For this review, use the dimensioned drawing (mm, ordinates from the lowest corner) and the shaded views. Round coordinates to 2 decimals unless told otherwise and drop trailing zeros. Order: outer loops, then holes, each group sorted by start corner. A loop starts at its lowest first (then second) coordinate and runs counter-clockwise, first axis right, second up. Notation, with made-up numbers: (-5, -36) - (14, -36) arc R21 ccw to (14, -24) - close; hole circle Ø1 at (46, 28.25). An arc over 180 degrees is marked (long way). Write item = value, one per line.
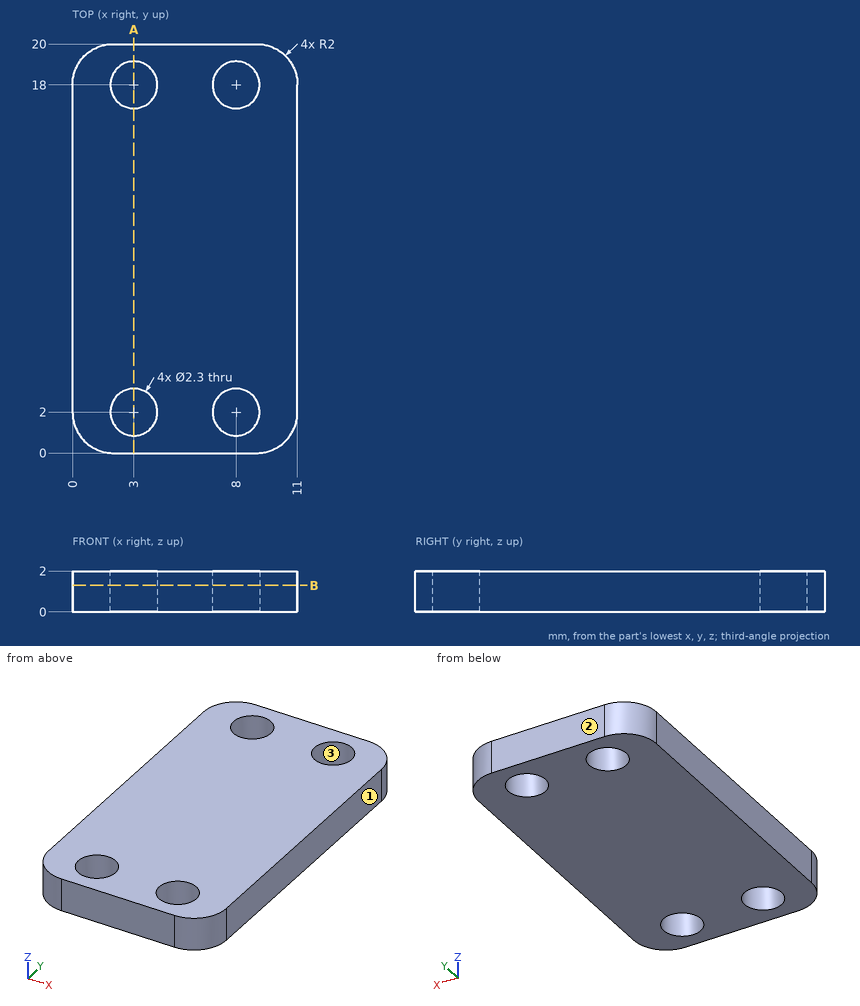
1) Clearance check with a flat-ended pin moving along its axis: pin 1 Ø1.8 at (x, y) = (8, 2) entering from +Z. State where the tip first meets the part, or that it passes through.
Findings:
pin_1 = through
2) To check wall thickness, follow L1, parallel to Y at x = 8, z = 0.8; L2, parallel to Y at x = 2.25, z = 0.1; L3, parallel to X at y = 1.5, z = 0.75. State the ranges of each line that lie inside material, in increasing order. Write a range as from..to.
Findings:
L1 = 0..0.85, 3.15..16.85, 19.15..20
L2 = 0..1.13, 2.87..17.13, 18.87..20
L3 = 0.06..1.96, 4.04..6.96, 9.04..10.94
3) The part is to be moulded in two halves that separate along Y. For the marked faces 1, 2 and 3, say which applies: released by +Y, released by -Y, zero draft, split by the parting line, or undercut.
Findings:
face_1 = zero draft
face_2 = released by +Y
face_3 = undercut
4) We need section B-B on z = 1.3. Write out the cut boundary in (x, y).
Findings:
outline = (0, 2) arc R2 ccw to (2, 0) - (9, 0) arc R2 ccw to (11, 2) - (11, 18) arc R2 ccw to (9, 20) - (2, 20) arc R2 ccw to (0, 18) - close; hole circle Ø2.3 at (3, 2); hole circle Ø2.3 at (3, 18); hole circle Ø2.3 at (8, 2); hole circle Ø2.3 at (8, 18)
5) We need section A-A on x = 3. Write out the cut boundary in (y, z), and give its area (3 significant figures).
Findings:
outline = (0, 0) - (0.85, 0) - (0.85, 2) - (0, 2) - close; (3.15, 0) - (16.85, 0) - (16.85, 2) - (3.15, 2) - close; (19.15, 0) - (20, 0) - (20, 2) - (19.15, 2) - close
area = 30.8 mm^2
